from build123d import *

# Parameters (mm, degrees)
SKETCH1_R                          = 19.05
BOSS_EXTRUDE1_DEPTH                = 57.15
SKETCH2_R                          = 15.875
CUT_EXTRUDE1_DEPTH                 = 53.975
SKETCH3_R                          = 6.35
CUT_EXTRUDE2_DEPTH                 = 48.26
F_1_16_0_0625_DIAMETER_HOLE1_D     = 1.5875
F_1_16_0_0625_DIAMETER_HOLE1_DEPTH = 13.97
CIRPATTERN1_COUNT                  = 3


with BuildPart() as part:
    # Sketch1 → Boss-Extrude1 (new body)
    with BuildSketch(Plane(origin=(0, 0, 0), x_dir=(1, 0, 0), z_dir=(0, 1, 0))):
        with Locations(Location((0.524325323, 0, 0), (0, 0, 270))):
            Circle(SKETCH1_R)
    extrude(amount=BOSS_EXTRUDE1_DEPTH)

    # Sketch2 → Cut-Extrude1 (cut)
    with BuildSketch(Plane(origin=(0, 57.15, 0), x_dir=(1, 0, 0), z_dir=(0, 1, 0))):
        with Locations(Location((0.524325323, 0, 0), (0, 0, 270))):
            Circle(SKETCH2_R)
    extrude(amount=-CUT_EXTRUDE1_DEPTH, mode=Mode.SUBTRACT)

    # Sketch3 → Cut-Extrude2 (cut)
    with BuildSketch(Plane(origin=(0, 0, 0), x_dir=(-1, 0, 0), z_dir=(0, -1, 0))):
        with Locations(Location((0, 0, 0), (0, 0, 90))):
            Circle(SKETCH3_R)
    extrude(amount=-CUT_EXTRUDE2_DEPTH, mode=Mode.SUBTRACT)

    # 1/16 (0.0625) Diameter Hole1
    with Locations(Plane(origin=(16.398633507, 54.077107179, 0.148204826), x_dir=(0.009335737046, 0, -0.999956421057), z_dir=(-0.999956421057, 0, -0.009335737046))):
        with Locations((0, 0)):
            f_1_16_0_0625_diameter_hole1 = Hole(F_1_16_0_0625_DIAMETER_HOLE1_D / 2, depth=F_1_16_0_0625_DIAMETER_HOLE1_DEPTH)

    # CirPattern1: 1/16 (0.0625) Diameter Hole1 ×3 about axis
    cirpattern1_axis = Axis((0.524325323, 57.15, 0), (0, -1, 0))
    for i in range(1, CIRPATTERN1_COUNT):
        add(f_1_16_0_0625_diameter_hole1.rotate(cirpattern1_axis, i * 360 / CIRPATTERN1_COUNT), mode=Mode.SUBTRACT)


solid = part.part
Source: CAD feature listing. Evaluate the final solid. Frame: model axes, mm. A direction names the side the tool comes from. Coordinates: 2 decimals unless noted, no trailing zeros. Loops run counter-clockwise (first coordinate to the right, second up) from the corner with the lowest first, then second, coordinate; pieces in that order, holes last. Notation, with made-up numbers: (26.25, -11) - (71.25, -11) arc R9 cw to (71.25, -6) - close; hole circle Ø10 at (46, 13). An arc over 180 degrees is marked (long way). One line per item, written item: value. Start each with the question number.
1. Ray query, L1, parallel to X at y = 1.6, z = 0; L2, parallel to X at y = 39, z = 0; L3, parallel to Z at x = 0, y = 49.5. Return the intervals inside material, ascending.
2. Set-up query: faces 1 (the flat face through (1, 3.175, 7)), 2 (the flat face through (5, 0, -5)). Return all of +Z, -Z, +X, -X, +Y, -Y with unobstructed straight access to the full face (end or side cutting, diameter ignored); none if empty.
3. Section D-D (y = 20.5). Return the cut outline in (x, z) (3 decimals), and give its area (3 significant figures).
4. Contact query for flat-ended pins moving along their axis: P1, Ø10, axis at x = 6.5, z = 5, coming from the +Y side (3 decimals); P2, Ø1, axis at y = 29, z = 5.5, coming from the +X side; P3, Ø10, axis at x = 15, y = 39, coming from the +Z side. Output: stop coordinate, or through.
5. Section B-B (x = -11). Return the cut outline in (y, z) (3 decimals).
6. Mould query, pull axis X, two halves, no side actions, for faces 3 (the cylindrical face through (-18.073, 28.175, -4.13)), 4 (the flat face through (15, 57.15, -7)), 5 (the cylindrical face through (-3.86, 1.57, 5.04)). Classes: pulls with the +X half, pulls with the -X half, needs draft (parallel to the pull), parting line crosses it, or undercut.
7. Section A-A (z = -5). Return the cut outline in (x, y) (3 decimals), and give its area (3 significant figures).
8. Section C-C (z = 0). State how many separate pieces and enclosed holes the cut face has, and give its area (3 significant figures).
Verdict:
1. L1: x = -18.53 to -6.35, 6.35 to 19.57
1. L2: x = -18.53 to -15.35, 16.4 to 19.57
1. L3: z = -19.04 to -15.87, 15.87 to 19.04
2. face 1: +Y
2. face 2: +Z, -Z, +X, -X, -Y
3. outline: circle Ø38.1 at (0.524, 0); hole circle Ø31.75 at (0.524, 0)
3. area: 348 mm2
4. P1: stops at y = 3.175
4. P2: stops at x = 18.91
4. P3: stops at z = 16.53
5. outline: (0, -15.169) - (57.15, -15.169) - (57.15, -10.918) - (3.175, -10.918) - (3.175, 10.918) - (57.15, 10.918) - (57.15, 15.169) - (0, 15.169) - close
6. face 3: parting line crosses it
6. face 4: needs draft
6. face 5: undercut
7. outline: (-17.858, 0) - (-3.914, 0) - (-3.914, 3.175) - (-14.543, 3.175) - (-14.543, 57.15) - (-17.858, 57.15) - close; (3.914, 0) - (18.906, 0) - (18.906, 57.15) - (15.591, 57.15) - (15.591, 3.175) - (3.914, 3.175) - close
7. area: 450 mm2
8. separate pieces: 3
8. enclosed holes: 0
8. area: 418 mm2
